```python
from build123d import *

# Parameters (mm, degrees)
BOSS_EXTRUDE1_DEPTH = 4.5
SKETCH2_W           = 10
SKETCH2_H           = 15.0114
BOSS_EXTRUDE2_DEPTH = 1.778
FILLET1_R           = 0.889
SKETCH3_W           = 3.7
SKETCH3_H           = 0.508
BOSS_EXTRUDE3_DEPTH = 4
FILLET2_R           = 0.5
SKETCH4_R           = 0.75
CUT_EXTRUDE1_DEPTH  = 12.5797
BOSS_EXTRUDE4_DEPTH = 3.15


with BuildPart() as part:
    # Sketch1 → Boss-Extrude1 (new body, symmetric)
    with BuildSketch(Plane(origin=(0, 0, 0), x_dir=(0, 0, -1), z_dir=(1, 0, 0))):
        Polygon((-5.75, 0), (-5.75, -8.0264), (5.75, -8.0264), (5.75, 0), (7.5057, 0), (7.5057, 1.778), (-7.5057, 1.778), (-7.5057, 0), align=None)
    extrude(amount=BOSS_EXTRUDE1_DEPTH, both=True)

    # Sketch2 → Boss-Extrude2 (add)
    with BuildSketch(Plane(origin=(0, 1.778, 0), x_dir=(1, 0, 0), z_dir=(0, 1, 0))):
        Rectangle(SKETCH2_W, SKETCH2_H)
    extrude(amount=-BOSS_EXTRUDE2_DEPTH)

    # Fillet1
    fillet1_edges = [part.edges().sort_by_distance(p)[0] for p in [
        (0, 1.778, 7.5057),
        (0, 1.778, -7.5057),
        (5, 0.889, 7.5057),
        (5, 1.778, 0),
        (5, 0.889, -7.5057),
        (-5, 0.889, 7.5057),
        (-5, 0.889, -7.5057),
        (-5, 1.778, 0),
    ]]
    fillet(fillet1_edges, radius=FILLET1_R)

    # Sketch3 → Boss-Extrude3 (add)
    with BuildSketch(Plane.XZ.offset(8.0264)):
        with Locations((0, 3.82)):
            Rectangle(SKETCH3_W, SKETCH3_H)
        with Locations((0, -0.68)):
            Rectangle(SKETCH3_W, SKETCH3_H)
    extrude(amount=BOSS_EXTRUDE3_DEPTH)

    # Fillet2
    fillet2_edges = [part.edges().sort_by_distance(p)[0] for p in [
        (1.85, -12.0264, 3.82),
        (-1.85, -12.0264, 3.82),
        (1.85, -12.0264, -0.68),
        (-1.85, -12.0264, -0.68),
    ]]
    fillet(fillet2_edges, radius=FILLET2_R)

    # Sketch4 → Cut-Extrude1 (cut, through all)
    with BuildSketch(Plane.XY.offset(4.074)):
        with Locations((0, -9.7764)):
            Circle(SKETCH4_R)
    extrude(amount=-CUT_EXTRUDE1_DEPTH, mode=Mode.SUBTRACT)

    # Sketch5 → Boss-Extrude4 (add, symmetric)
    with BuildSketch(Plane(origin=(0, 0, 0), x_dir=(0, 0, -1), z_dir=(1, 0, 0))):
        with BuildLine():
            Line((4.734, 1.778), (-4.028021931, 3.690536137))
            ThreePointArc((-4.028021931, 3.690536137), (-4.179670828, 3.676927945), (-4.29629138, 3.579039143))
            ThreePointArc((-4.29629138, 3.579039143), (-4.807252645, 2.698529173), (-5.242, 1.778))
            Line((-5.242, 1.778), (4.734, 1.778))
        make_face()
    extrude(amount=BOSS_EXTRUDE4_DEPTH, both=True)


solid = part.part
```
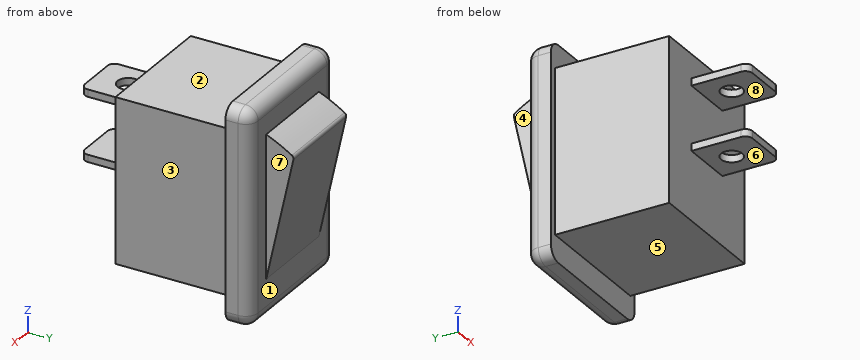
CAD build for the part. Positions are in the model's coordinates, mm. Face numbers are marked on the shaded views. A direction names the side the tool comes from. Coordinates: 2 decimals unless noted, no trailing zeros. Order: outer loops, then holes, each group sorted by start corner. A loop starts at its lowest first (then second) coordinate and runs counter-clockwise, first axis right, second up. Notation, with made-up numbers: (-35, 27) - (18, 27) arc R19 ccw to (18, 33) - close; hole circle Ø6 at (38, 51.25). An arc over 180 degrees is marked (long way). Use a Markdown table: item, result. Add a question column.
(1) Saw through at C-C (z = -5). Give the cut face in (x, y).
(2) Saw through at D-D (z = 0.5). Give the cut face in (x, y), then the cut area to 3 significant figures.
(3) Which spindle directions (+Z, -Z, +X, -X, +Y, -Y) get a long thin tool onto all of the face, cutting with end or side? Do the marked faces 1, 2, 3, 4 and 5. Say none if no direction does.
(4) Pull direction Z, two halves, no side cores. Call the marked faces 6, 7 and 8: +Z half, -Z half, draft (parallel to the pull), parting line (faces both ways), or undercut.
(5) Saw through at A-A (y = -8.5). Give the cut face in (x, z).
(6) Drill centre lines: line 1 along X through (y, z) = (-7.5, 4.5); line 2 along Z through (x, y) = (1.5, -9.5); line 3 along Z through (x, y) = (-1.75, -3.75). Where is each one in solid material? Low to high. Write a range as [from, to].
(7) Saw through at B-B (x = 0). Count the separate pieces of the cut face and the enclosed holes in it, then the cut area to 3 significant figures.
(8) Flat gauge pins, fed straight in: pin 1 (2.5 mm diameter, centred on y = -5.5, z = -1, fed in from -X); pin 2 (1.5 mm diameter, centred on y = -8, z = -5.5, fed in from +X); pin 3 (0.6 mm diameter, centred on y = -10.5, z = -0.5, fed in from -X). Where does each tip first touch, or does it go through?
Solved:
| question | item | result |
|---|---|---|
| 1 | outline | (-5, 0) - (-4.5, 0) - (-4.5, -8.03) - (4.5, -8.03) - (4.5, 0) - (5, 0) - (5, 0.89) arc R0.89 ccw to (4.11, 1.78) - (-4.11, 1.78) arc R0.89 ccw to (-5, 0.89) - close |
| 2 | outline | (-5, 0) - (-4.5, 0) - (-4.5, -8.03) - (4.5, -8.03) - (4.5, 0) - (5, 0) - (5, 0.89) arc R0.89 ccw to (4.11, 1.78) - (3.15, 1.78) - (3.15, 2.92) - (-3.15, 2.92) - (-3.15, 1.78) - (-4.11, 1.78) arc R0.89 ccw to (-5, 0.89) - close |
| 2 | area | 96.9 mm² |
| 3 | face 1 | +Y |
| 3 | face 2 | +Z, +X, -X, -Y |
| 3 | face 3 | +Z, -Z, +X, -Y |
| 3 | face 4 | +Z, -Z, -X, +Y |
| 3 | face 5 | -Z, +X, -X, -Y |
| 4 | face 6 | -Z half |
| 4 | face 7 | draft |
| 4 | face 8 | undercut |
| 5 | outline | (-1.85, -0.93) - (1.85, -0.93) - (1.85, -0.43) - (-1.85, -0.43) - close; (-1.85, 3.57) - (1.85, 3.57) - (1.85, 4.07) - (-1.85, 4.07) - close |
| 6 | line 1 | x = [-4.5, 4.5] |
| 6 | line 2 | z = [-0.93, -0.43], [3.57, 4.07] |
| 6 | line 3 | z = [-5.75, 5.75] |
| 7 | separate pieces | 3 |
| 7 | enclosed holes | 0 |
| 7 | area | 131 mm² |
| 8 | pin 1 | stops at x = -4.5 |
| 8 | pin 2 | stops at x = 4.5 |
| 8 | pin 3 | stops at x = -1.85 |
